from build123d import *

# Parameters (mm, degrees)
SKETCH1_R           = 1.905
BOSS_EXTRUDE1_DEPTH = 8.89
SKETCH2_W           = 6.35
SKETCH2_H           = 6.35
BOSS_EXTRUDE2_DEPTH = 2.54


with BuildPart() as part:
    # Sketch1 → Boss-Extrude1 (new body)
    with BuildSketch(Plane.XY):
        Circle(SKETCH1_R)
    extrude(amount=-BOSS_EXTRUDE1_DEPTH)

    # Sketch2 → Boss-Extrude2 (add)
    with BuildSketch(Plane.XY):
        Rectangle(SKETCH2_W, SKETCH2_H)
    extrude(amount=BOSS_EXTRUDE2_DEPTH)


solid = part.part
Here's how the part is built. I have some questions about the finished solid (model axes, mm). A direction names the side the tool comes from. Coordinates: 2 decimals unless noted, no trailing zeros. Write each loop counter-clockwise with the first axis right and the second up, starting at its lowest first coordinate (ties: lowest second). Pieces come first, ordered by that corner, then holes.
Item 1: I want a section at A-A on x = 0. Write out the boundary of the cut face in (y, z) (3 decimals), and give its area (3 significant figures).
Item 2: If I drill on line 1 (Z direction, x = 2.25, y = -0.75); line 2 (Y direction, x = 0, z = -4.5) (3 decimals); line 3 (X direction, y = 0.5, z = -1.5), over which ranges is the centre line in solid material (lowest first)?
Item 3: I want a section at B-B on y = -1. Write out the boundary of the cut face in (x, z) (3 decimals).
Item 4: On a 3-axis mill with a long thin cutter (end or side, diameter ignored), from which of +Z, -Z, +X, -X, +Y, -Y can I reach the whole of each face in a straight line? I mean faces 1 (the flat face through (-1.5, 1.5, 0)), 2 (the flat face through (-3.175, 0, 1)). Say none if no direction works.
Item 5: Will these pins go through, and if not, where does the flat tip stop? pin 1 (1 mm diameter, centred on x = -2.5, y = -2, fed in from -Z); pin 2 (1.5 mm diameter, centred on x = 0.5, z = -6.5, fed in from +Y) (3 decimals); pin 3 (2 mm diameter, centred on x = -1.5, z = -3, fed in from -Y).
Item 6: I want a section at D-D on x = -2.5. Write out the boundary of the cut face in (y, z) (3 decimals).
Item 7: I want a section at C-C on z = -2.5. Write out the boundary of the cut face in (x, y) (3 decimals).
Findings below:
1. outline: (-3.175, 0) - (-1.905, 0) - (-1.905, -8.89) - (1.905, -8.89) - (1.905, 0) - (3.175, 0) - (3.175, 2.54) - (-3.175, 2.54) - close
1. area: 50.0 mm2
2. line 1: z = 0 to 2.54
2. line 2: y = -1.905 to 1.905
2. line 3: x = -1.84 to 1.84
3. outline: (-3.175, 0) - (-1.621, 0) - (-1.621, -8.89) - (1.621, -8.89) - (1.621, 0) - (3.175, 0) - (3.175, 2.54) - (-3.175, 2.54) - close
4. face 1: -Z
4. face 2: +Z, -Z, -X, +Y, -Y
5. pin 1: stops at z = 0
5. pin 2: stops at y = 1.905
5. pin 3: stops at y = -1.84
6. outline: (-3.175, 0) - (3.175, 0) - (3.175, 2.54) - (-3.175, 2.54) - close
7. outline: circle Ø3.81 at (0, 0)
